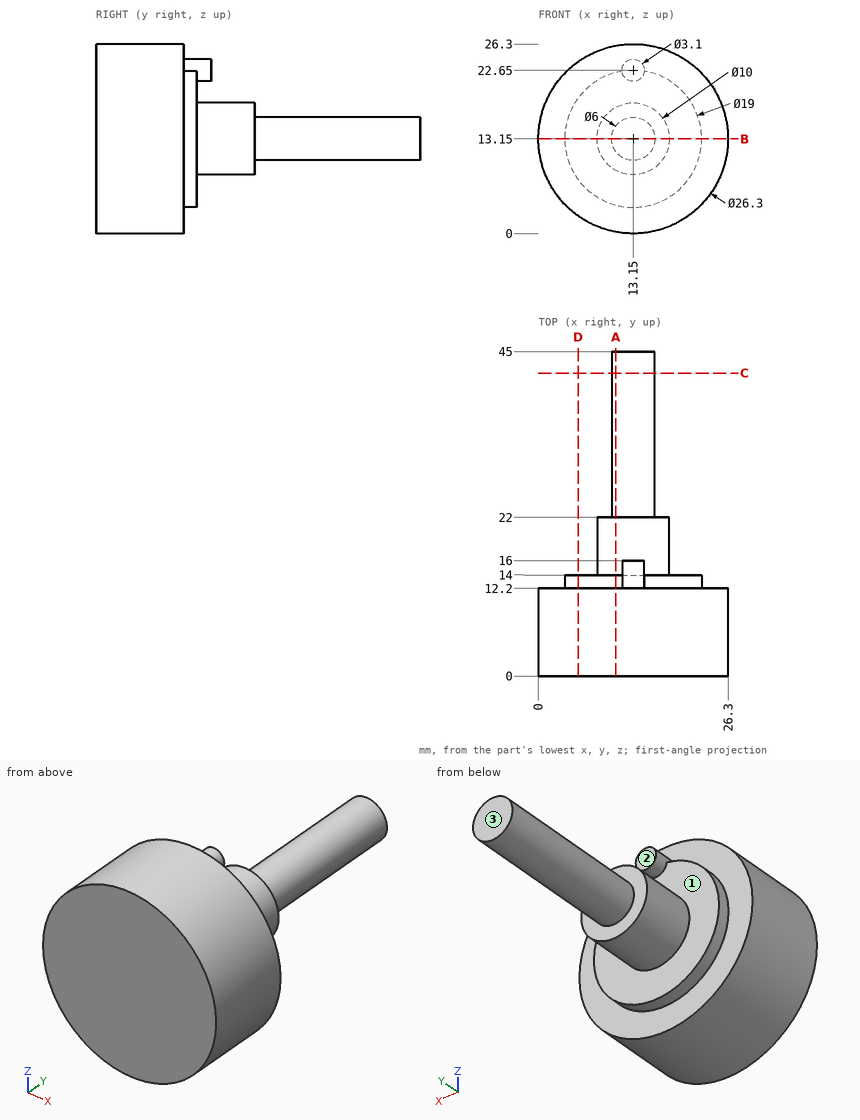
Here's the drawing with two shaded views (mm, measured from the low corner). I have some questions. A direction names the side the tool comes from. Coordinates: 2 decimals unless noted, no trailing zeros. Write each loop counter-clockwise with the first axis right and the second up, starting at its lowest first coordinate (ties: lowest second). Pieces come first, ordered by that corner, then holes. Notation, with made-up numbers: (-16.75, 8.5) -> (-9.75, 8.5) arc R35 ccw to (-9.75, 41.5) -> close; hole circle Ø1 at (-39.75, 24). An arc over 180 degrees is marked (long way). One line per question, with ' | ' between items. Start each with the question number.
1. If we section it at B-B (z = 13.15): Please give me the cut outline in (x, y).
2. If we section it at D-D (x = 5.5): Please give me the cut outline in (y, z).
3. For the marked faces 1, 2 and 3, which set-ups out of +Z, -Z, +X, -X, +Y, -Y let a thin tool reach every point of the face, with its end or its side?
4. If we section it at C-C (y = 42): Please give me the cut outline in (x, z).
5. If we section it at A-A (x = 10.75): Please give me the cut outline in (y, z).
6. Please list where these lines run through material, in increasing order: line 1 along Y through (x, z) = (3.25, 16); line 2 along Y through (x, z) = (11.25, 6); line 3 along X through (y, z) = (18.5, 13).
7. Will these pins go through, and if not, where does the flat tip stop? P1, Ø2, axis at x = 5.5, z = 3, coming from the +Y side; P2, Ø10, axis at y = 33.5, z = 17, coming from the -X side; P3, Ø1.6, axis at x = 13, z = 23, coming from the +Y side.
Return value:
1) outline: (0, 0) -> (26.3, 0) -> (26.3, 12.2) -> (22.65, 12.2) -> (22.65, 14) -> (18.15, 14) -> (18.15, 22) -> (16.15, 22) -> (16.15, 45) -> (10.15, 45) -> (10.15, 22) -> (8.15, 22) -> (8.15, 14) -> (3.65, 14) -> (3.65, 12.2) -> (0, 12.2) -> close
2) outline: (0, 2.45) -> (12.2, 2.45) -> (12.2, 7.52) -> (14, 7.52) -> (14, 18.78) -> (12.2, 18.78) -> (12.2, 23.85) -> (0, 23.85) -> close
3) face 1: +Y | face 2: +Z, +X, -X, +Y | face 3: +Z, -Z, +X, -X, +Y
4) outline: circle Ø6 at (13.15, 13.15)
5) outline: (0, 0.22) -> (12.2, 0.22) -> (12.2, 3.96) -> (14, 3.96) -> (14, 8.76) -> (22, 8.76) -> (22, 11.35) -> (45, 11.35) -> (45, 14.95) -> (22, 14.95) -> (22, 17.54) -> (14, 17.54) -> (14, 22.34) -> (12.2, 22.34) -> (12.2, 26.08) -> (0, 26.08) -> close
6) line 1: y = 0 to 12.2 | line 2: y = 0 to 14 | line 3: x = 8.15 to 18.15
7) P1: stops at y = 12.2 | P2: stops at x = 10.15 | P3: stops at y = 16
